The model under review builds one solid part; all positions refer to its coordinate system, in mm. Face numbers are marked on the shaded views. Coordinates: 2 decimals unless noted, no trailing zeros. Order: outer loops, then holes, each group sorted by start corner. A loop starts at its lowest first (then second) coordinate and runs counter-clockwise, first axis right, second up. Notation, with made-up numbers: M 32,-30.75 L 68,-30.75 A21 cw 68,4.25 Z; hole C 13,88 d3. An arc over 180 degrees is marked long. Write each question's results on one line, items separated by ' | '.
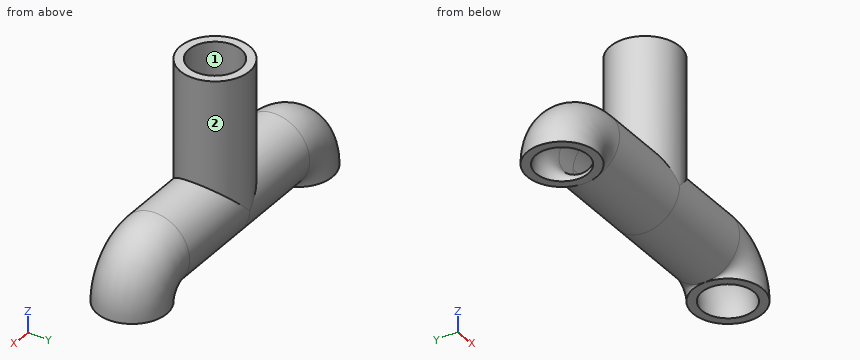
from build123d import *
from build123d import SkipClean  # not in build123d's __all__

# Parameters (mm, degrees)
F0_R      = 1
F0_R_2    = 0.75
F4_DEPTH  = 2.61254
F5_DEPTH  = 2.61254
F8_R      = 1
F8_R_2    = 0.75
F9_DEPTH  = 4
F10_R     = 0.75
F11_DEPTH = 4
F13_R     = 0.75
F14_DEPTH = 4


# Not quite as in the source:
# - after a boolean that leaves OpenCascade's solid faulty, fix() repairs it


with BuildPart() as f2:
    # F2: sweep along a path in F1
    with BuildLine(Plane.XZ) as f2_path:
        ThreePointArc((-2.61254, 1), (-3.3196467812, 0.7071067812), (-3.61254, 0))
    # F0 (on Top) → F2 (sweep)
    with BuildSketch(Plane.XY):
        with Locations((-3.61254, 0)):
            Circle(F0_R)
        with Locations((-3.61254, 0)):
            Circle(F0_R_2, mode=Mode.SUBTRACT)
    sweep(path=f2_path.line)

    # F5 (add): a face of the model
    f5_faces = [f2.faces().sort_by_distance(p)[0] for p in [
        (-2.61254, 0, 1.9717157288),
    ]]


with BuildPart() as f3:
    # F3: sweep along a path in F1
    with BuildLine(Plane.XZ) as f3_path:
        ThreePointArc((2.61254, 1), (3.3196467812, 0.7071067812), (3.61254, 0))
    # F0 (on Top) → F3 (sweep)
    with BuildSketch(Plane.XY):
        with BuildLine():
            ThreePointArc((4.61254, 0), (3.61254, 1), (2.61254, 0))
            ThreePointArc((2.61254, 0), (3.61254, -1), (4.61254, 0))
        make_face()
        with BuildLine():
            ThreePointArc((4.36254, 0), (3.61254, -0.75), (2.86254, 0))
            ThreePointArc((2.86254, 0), (3.61254, 0.75), (4.36254, 0))
        make_face(mode=Mode.SUBTRACT)
    sweep(path=f3_path.line)

    # F4 (add): a face of the model
    f4_faces = [f3.faces().sort_by_distance(p)[0] for p in [
        (2.61254, 0.9717157288, 1),
    ]]
    extrude(f4_faces, amount=F4_DEPTH)


with BuildPart() as f2_1:
    add(f2.part, clean=False)

    add(f3.part)  # F5 merges F3
    extrude(f5_faces, amount=F5_DEPTH)

    # F6: union 

    # F8 (on offset) → F9 (join)
    with BuildSketch(Plane.XY.offset(1)):
        Circle(F8_R)
        Circle(F8_R_2, mode=Mode.SUBTRACT)
    with SkipClean():  # cleaning this boolean's faces spoils the solid; the shape is the same uncleaned
        extrude(amount=F9_DEPTH)

    # F10 (on face) → F11 (cut)
    with BuildSketch(Plane.XY.offset(5)):
        Circle(F10_R)
    extrude(amount=-F11_DEPTH, mode=Mode.SUBTRACT)

    add(f2_1.part.fix(), mode=Mode.REPLACE)

    # F13 (on offset) → F14 (cut)
    with BuildSketch(Plane.YZ.offset(2)):
        with Locations((0, 1)):
            Circle(F13_R)
    extrude(amount=-F14_DEPTH, mode=Mode.SUBTRACT)


solid = f2_1.part
1) Take a section at A-A on x = -1.75. State the section outline as (y, z) points.
Solutions:
outline: C 0,1 d2; hole C 0,1 d1.5
2) Take a section at D-D on x = 0.5. State the section outline as (y, z) points, plus the area to 3 significant figures.
Solutions:
outline: M -0.87,1.5 A1 ccw long 0.87,1.5 L 0.87,5 L 0.56,5 L 0.56,1.5 A0.75 cw long -0.56,1.5 L -0.56,5 L -0.87,5 Z | area: 3.10 mm2
3) For pin 1 (1.2 mm diameter, centred on y = 0, z = 1, fed in from +X); pin 2 (1.2 mm diameter, centred on y = 0, z = 1, fed in from -X); pin 3 (1 mm diameter, centred on y = 0.5, z = 2, fed in from -X), all flat-tipped, find the tip position at first contact; note any pin that passes through.
Solutions:
pin 1: x = 4.57 | pin 2: x = -4.57 | pin 3: x = -3.81
4) Take a section at C-C on z = 2.6. State the section outline as (x, y) points, plus the area to 3 significant figures.
Solutions:
outline: C 0,0 d2; hole C 0,0 d1.5 | area: 1.37 mm2
5) Take a section at B-B on y = -0.35. Count the separate pieces of the cut face and the enclosed holes in it, plus the area to 3 significant figures.
Solutions:
separate pieces: 3 | enclosed holes: 0 | area: 5.89 mm2
6) To check wall thickness, follow line 1 along Y through (x, z) = (1.2, 1); line 2 along Z through (x, y) = (-2, -0.6). State the ranges of each line that lie inside material, in increasing order.
Solutions:
line 1: -1 to -0.75, 0.75 to 1 | line 2: 0.2 to 0.55, 1.45 to 1.8
7) The part is to be moulded in two halves that separate along Y. For the marked faces 1 and 2, say which applies: pulls with the +Y half, pulls with the -Y half, needs draft (parallel to the pull), parting line crosses it, or undercut.
Solutions:
face 1: undercut | face 2: parting line crosses it
